Source: CAD feature listing. Evaluate the final solid. Frame: model axes, mm. Coordinates: 2 decimals unless noted, no trailing zeros. Write each loop counter-clockwise with the first axis right and the second up, starting at its lowest first coordinate (ties: lowest second). Pieces come first, ordered by that corner, then holes. Notation, with made-up numbers: (-12.5, 37) - (37.5, 37) arc R17 ccw to (37.5, 56) - close; hole circle Ø10 at (83.5, -38). An arc over 180 degrees is marked (long way). One line per question, with ' | ' between items.
Autodesk Inventor part; units mm, degrees
ref_plane "YZ Plane" through (0, 0, 0) normal (1, 0, 0) x (0, 1, 0)
ref_plane "XZ Plane" through (0, 0, 0) normal (0, 1, 0) x (-1, 0, 0)
ref_plane "XY Plane" through (0, 0, 0) normal (0, 0, 1) x (1, 0, 0)
sketch "草圖1" plane through (0, 0, 0) normal (0, 0, 1) x (1, 0, 0)
  line L0 (-120, 0) -> (0, 0) construction
  line L1 (-120, -5) -> (0, -5)
  line L2 (0, 5) -> (-120, 5)
  arc A0 (-120, 5) -> (-120, -5) centre (-120, 0) ccw
  arc A1 (0, -5) -> (0, 5) centre (0, 0) ccw
  circle A2 centre (-120, 0) radius 2.1
  circle A3 centre (0, 0) radius 2.1
  circle A4 centre (-110, 0) radius 2.1
  circle A5 centre (-100, 0) radius 1.6
  circle A6 centre (-90, 0) radius 1.6
  circle A7 centre (-80, 0) radius 1.6
  circle A8 centre (-70, 0) radius 1.6
  circle A9 centre (-60, 0) radius 1.6
  circle A10 centre (-50, 0) radius 1.6
  circle A11 centre (-40, 0) radius 1.6
  circle A12 centre (-30, 0) radius 1.6
  circle A13 centre (-20, 0) radius 1.6
  circle A14 centre (-10, 0) radius 1.6
  dimension "d0" = 120
  dimension "d1" = 10
  dimension "d2" = 4.2
  dimension "d3" = 4.2
  dimension "d4" = 4.2
  dimension "d11" = 3.2
  dimension "d12" = 10
  dimension "d13" = 10
  dimension "d16" = 10
extrude "擠出1" add sketch "草圖1" along normal blind 3 contours A0 L2 A1 L1 | A5 | A6 | A7 | A8 | A9 | A10 | A11 | A12 | A13 | A14
extrude "擠出2" cut sketch "草圖1" along normal blind 10 contours A5 | A6 | A7 | A8 | A9 | A10 | A11 | A12 | A13 | A14
sketch "草圖3" plane through (0, 0, 3) normal (0, 0, 1) x (1, 0, 0)
  circle A0 centre (-10, 0) radius 1.6
  circle A1 centre (-50, 0) radius 1.6
  circle A2 centre (-80, 0) radius 1.6
  circle A3 centre (-40, 0) radius 1.6
  circle A4 centre (-90, 0) radius 1.6
  circle A5 centre (-20, 0) radius 1.6
  circle A6 centre (-60, 0) radius 1.6
  circle A7 centre (-70, 0) radius 1.6
  circle A8 centre (-30, 0) radius 1.6
  circle A9 centre (-100, 0) radius 1.6
  arc A10 (0, -5) -> (0, 5) centre (0, 0) ccw
  line L0 (0, 5) -> (-120, 5)
  arc A11 (-120, 5) -> (-120, -5) centre (-120, 0) ccw
  line L1 (-120, -5) -> (0, -5)
  circle A12 centre (0, 0) radius 2.1
  circle A13 centre (-110, 0) radius 2.1
  circle A14 centre (-120, 0) radius 2.1
properties part number "adjustable"
Item 1: Ray query, line 1 along Y through (x, z) = (-70, 1.55); line 2 along Y through (x, z) = (-120, 0.95); line 3 along X through (y, z) = (3, 1.55). Return the intervals inside material, ascending. Write a range as [from, to].
Check sheet entries:
line 1: [-5, -1.6], [1.6, 5] | line 2: [-5, -2.1], [2.1, 5] | line 3: [-124, 4]
Item 2: Cut plane C-C on x = -110. Return loops of the section in (y, z), and give its area (3 significant figures).
Check sheet entries:
outline: (-5, 0) - (-2.1, 0) - (-2.1, 3) - (-5, 3) - close; (2.1, 0) - (5, 0) - (5, 3) - (2.1, 3) - close | area: 17.4 mm²
Item 3: Mould query, pull axis Y, two halves, no side actions, for faces 1 (the face through (-112.1, -0.09, 1.48)), 2 (the face through (-59, 5, 1)), 3 (the face through (-61, 2, 0)). Classes: pulls with the +Y half, pulls with the -Y half, needs draft (parallel to the pull), parting line crosses it, or undercut.
Check sheet entries:
face 1: undercut | face 2: pulls with the +Y half | face 3: needs draft
Item 4: Cut plane B-B on z = 2.35. State how many separate pieces and enclosed holes the cut face has, and give its area (3 significant figures).
Check sheet entries:
separate pieces: 1 | enclosed holes: 13 | area: 1,160 mm²
Item 5: Cut plane A-A on x = -50. Return loops of the section in (y, z).
Check sheet entries:
outline: (-5, 0) - (-1.6, 0) - (-1.6, 3) - (-5, 3) - close; (1.6, 0) - (5, 0) - (5, 3) - (1.6, 3) - close
Item 6: Cut plane D-D on y = 3.75. Return loops of the section in (x, z).
Check sheet entries:
outline: (-123.31, 0) - (3.31, 0) - (3.31, 3) - (-123.31, 3) - close
Item 7: Pin query (flat end, axial travel): pin 1 Ø3 at (x, y) = (-90, 0) entering from +Z; pin 2 Ø1.5 at (y, z) = (2, 2.5) entering from -X. Return the tip coordinate at first contact, or that it passes through.
Check sheet entries:
pin 1: through | pin 2: x = -124.84
